from build123d import *

# Parameters (mm, degrees)
F0_W      = 118.301205337
F0_H      = 59.3464635313
F1_DEPTH  = 50.8
F2_W      = 52.4965906516
F2_H      = 14.247585088
F3_DEPTH  = 112.014
F4_W      = 50.1409089193
F4_H      = 6.169681903
F5_DEPTH  = 123.19
F7_DEPTH  = 96.52
F8_W      = 15.2773074806
F8_H      = 5.2911678412
F9_DEPTH  = 203.962
F10_R     = 4.445
F11_DEPTH = 210.566


with BuildPart() as f1:
    # F0 (on Top) → F1 (new body)
    with BuildSketch(Plane.XY):
        Rectangle(F0_W, F0_H)
    extrude(amount=F1_DEPTH)

    # F2 (on face) → F3 (cut)
    with BuildSketch(Plane.XY.offset(50.8)):
        with Locations((37.6030090265, -22.5494392216)):
            Rectangle(F2_W, F2_H)
    extrude(amount=-F3_DEPTH, mode=Mode.SUBTRACT)

    # F4 (on face) → F5 (cut)
    with BuildSketch(Plane.XZ.offset(29.6732317656)):
        with Locations((-34.0801482089, 3.0848409515)):
            Rectangle(F4_W, F4_H)
    extrude(amount=-F5_DEPTH, mode=Mode.SUBTRACT)

    # F6 (on face) → F7 (cut)
    with BuildSketch(Plane.XZ.offset(29.6732317656)):
        Polygon((11.3547137007, 50.8), (0, 50.8), (11.3547137007, 41.1124470571), align=None)
        Polygon((11.3547137007, 50.8), (11.3547137007, 41.1124470571), (59.5423281193, 0), (59.5423281193, 50.8), align=None)
    extrude(amount=-F7_DEPTH, mode=Mode.SUBTRACT)

    # F8 (on face) → F9 (cut)
    with BuildSketch(Plane(origin=(-59.1506026685, 0, 0), x_dir=(0, -1, 0), z_dir=(-1, 0, 0))):
        with Locations((0, 48.1544160794)):
            Rectangle(F8_W, F8_H)
    extrude(amount=-F9_DEPTH, mode=Mode.SUBTRACT)

    # F10 (on face) → F11 (cut)
    with BuildSketch(Plane(origin=(-59.1506026685, 0, 0), x_dir=(0, -1, 0), z_dir=(-1, 0, 0))):
        with Locations((-18.4111148119, 36.9201600552)):
            Circle(F10_R)
        with Locations((7.0510655642, 36.9201600552)):
            Circle(F10_R)
        with Locations((7.0510655642, 14.2000615597)):
            Circle(F10_R)
        with Locations((-18.4111148119, 14.2000615597)):
            Circle(F10_R)
    extrude(amount=-F11_DEPTH, mode=Mode.SUBTRACT)


solid = f1.part
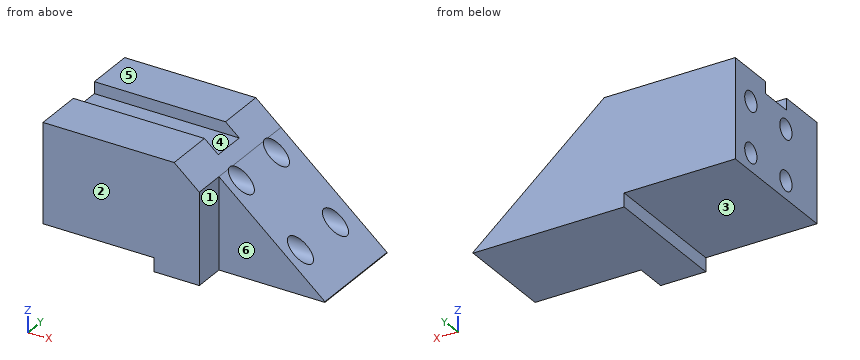
Could you check a few things on this model? Use its own coordinates, in mm. Face numbers are marked on the shaded views. A direction names the side the tool comes from. Round coordinates to 2 decimals unless told otherwise and drop trailing zeros. Write each loop counter-clockwise with the first axis right and the second up, starting at its lowest first coordinate (ties: lowest second). Pieces come first, ordered by that corner, then holes. Notation, with made-up numbers: (29.5, 45) - (76.5, 45) arc R29 ccw to (76.5, 73) - close; hole circle Ø11 at (-13, -11.75). An arc over 180 degrees is marked (long way). Put each result on its own line as item: value. Start each with the question number.
(1) Thinking about a two-plate mould opening in Y: for the marked faces 4, 5 and 6, which applies, released by +Y, released by -Y, zero draft, split by the parting line, or undercut?
(2) I want a section at D-D, the plane y = 12.5. Please give me the cut outline in (x, z).
(3) I want a section at B-B, the plane y = -4. Please give me the cut outline in (x, z), plus the area to 3 significant figures.
(4) I want a section at C-C, the plane x = 13.5. Please give me the cut outline in (y, z) (3 decimals).
(5) I need wall thicknesses on probe 1 along Z at (x, y) = (-7.5, -7); probe 2 along Z at (x, y) = (-2.5, 18); probe 3 along Y at (x, z) = (38, 14). Which ranges of each line are inside material? Lowest first, please.
(6) I want a section at A-A, the plane z = 17. Please give me the cut outline in (x, y), plus the area to 3 significant figures.
(7) For the marked faces 1, 2 and 3, which set-ups out of +Z, -Z, +X, -X, +Y, -Y let a thin tool reach every point of the face, with its end or its side?
(8) Will these pins go through, and if not, where does the flat tip stop? pin 1 (7 mm diameter, centred on y = -9.5, z = 2.5, fed in from -X); pin 2 (8 mm diameter, centred on y = 22.5, z = 14, fed in from +X); pin 3 (12 mm diameter, centred on x = -22, y = 0.5, fed in from +Z).
Here are the results:
1. face 4: undercut
1. face 5: zero draft
1. face 6: released by -Y
2. outline: (-59.15, 6.17) - (-9.01, 6.17) - (-9.01, 0) - (59.15, 0) - (59.15, 0.33) - (0, 50.8) - (-59.15, 50.8) - close
3. outline: (-59.15, 6.17) - (-9.01, 6.17) - (-9.01, 0) - (59.15, 0) - (59.15, 0.33) - (46.69, 10.97) - (-59.15, 10.97) - close; (-59.15, 17.43) - (39.11, 17.43) - (20.06, 33.69) - (-59.15, 33.69) - close; (-59.15, 40.15) - (12.48, 40.15) - (6.2, 45.51) - (-59.15, 45.51) - close
3. area: 2,730 mm^2
4. outline: (-15.426, 0) - (29.673, 0) - (29.673, 39.282) - (22.177, 39.282) arc R4.445 cw (long way) to (14.646, 39.282) - (-3.286, 39.282) arc R4.445 cw (long way) to (-10.817, 39.282) - (-15.426, 39.282) - close; hole circle Ø8.89 at (-7.051, 14.2); hole circle Ø8.89 at (18.411, 14.2)
5. probe 1: z = 0 to 9.76, 18.64 to 32.48, 41.36 to 45.51
5. probe 2: z = 0 to 9.77, 18.63 to 32.49, 41.35 to 50.8
5. probe 3: y = -15.43 to -11.49, -2.61 to 13.97, 22.85 to 29.67
6. outline: (-59.15, -29.67) - (11.35, -29.67) - (11.35, -15.43) - (39.62, -15.43) - (39.62, -10.5) - (-59.15, -10.5) - close; (-59.15, -3.6) - (39.62, -3.6) - (39.62, 14.96) - (-59.15, 14.96) - close; (-59.15, 21.86) - (39.62, 21.86) - (39.62, 29.67) - (-59.15, 29.67) - close
6. area: 4,090 mm^2
7. face 1: +Z, -Z, +X, -Y
7. face 2: +Z, -Z, +X, -X, -Y
7. face 3: -Z, -X, +Y, -Y
8. pin 1: stops at x = -9.01
8. pin 2: stops at x = 47.82
8. pin 3: stops at z = 45.51
